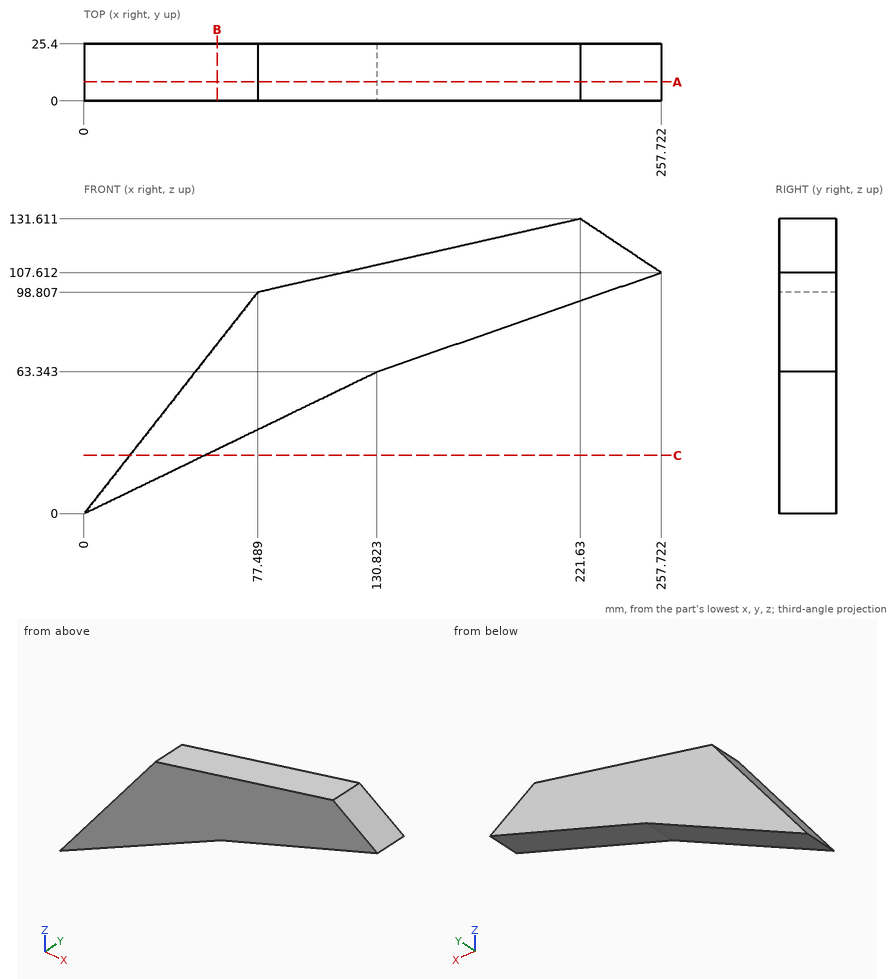
Design review of the part shown in the three views and the two pictorial views. Dimensions are in mm from the part's minimum x, y and z. Give positions to 0.01 mm unless a question says otherwise; leave off trailing zeros. Loops run counter-clockwise (first coordinate to the right, second up) from the corner with the lowest first, then second, coordinate; pieces in that order, holes last. Notation, with made-up numbers: M 22,33.5 L 29,33.5 A18 ccw 29,56.5 Z; hole C 53,53 d3. An arc over 180 degrees is marked long. Answer as a JSON object with one key per item and string values.
Item 1: For P1, Ø2, axis at x = 122, y = 15.5, coming from the -Z side; P2, Ø1.5, axis at x = 48, y = 4.5, coming from the +Z side; P3, Ø1.5, axis at y = 10, z = 14.5, coming from the -X side (1 decimal), all flat-tipped, find the tip position at first contact; note any pin that passes through.
Output values:
{"P1": "stops at z = 58.59", "P2": "stops at z = 62.16", "P3": "stops at x = 10.8"}
Item 2: We need section B-B (x = 59.5). State the section outline as (y, z) points.
Output values:
{"outline": "M 0,28.81 L 25.4,28.81 L 25.4,75.87 L 0,75.87 Z"}
Item 3: We need section A-A (y = 8.5). State the section outline as (x, z) points.
Output values:
{"outline": "M 0,0 L 130.82,63.34 L 257.72,107.61 L 221.63,131.61 L 77.49,98.81 Z"}
Item 4: Wall thickness on line 1 along X through (y, z) = (9.25, 32) (1 decimal); line 2 along X through (y, z) = (10, 16.5) (1 decimal); line 3 along Z through (x, y) = (115, 4.5) (1 decimal): over which ranges is each line inside the solid? List them lowest first.
Output values:
{"line 1": "x = 25.1 to 66.1", "line 2": "x = 12.9 to 34.1", "line 3": "z = 55.7 to 107.3"}
Item 5: We need section C-C (z = 26). State the section outline as (x, y) points, and give its area (3 significant figures).
Output values:
{"outline": "M 20.39,0 L 53.7,0 L 53.7,25.4 L 20.39,25.4 Z", "area": "846 mm2"}
